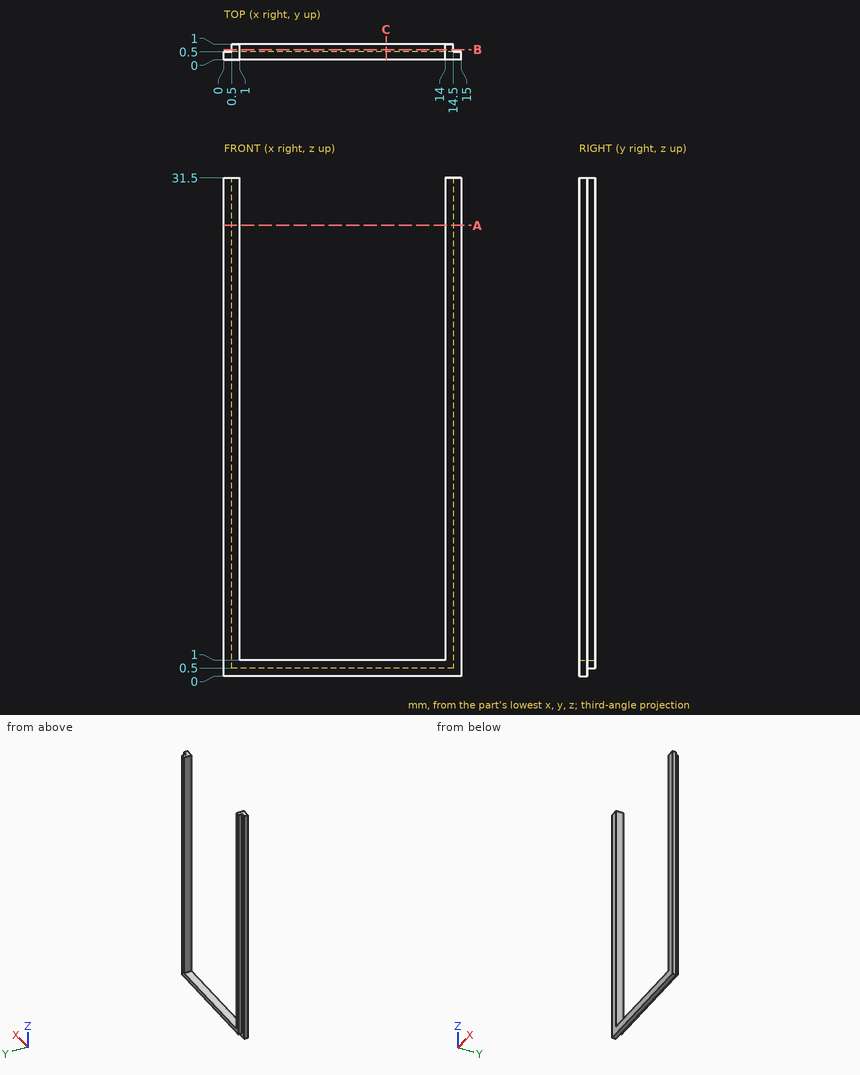
For this review, use the dimensioned drawing (mm, ordinates from the lowest corner) and the shaded views. Give positions to 0.01 mm unless a question says otherwise; leave off trailing zeros. Write each loop counter-clockwise with the first axis right and the second up, starting at its lowest first coordinate (ties: lowest second). Pieces come first, ordered by that corner, then holes.
(1) Consider section C-C, the plane x = 10.25. Give the boundary of the cut face in (y, z).
(2) To check wall thickness, follow L1, parallel to X at y = 0.55, z = 13; L2, parallel to X at y = 0.2, z = 13; L3, parallel to Z at x = 13.25, y = 0.3. State the ranges of each line that lie inside material, in increasing order.
(3) For P1, Ø0.6, axis at y = 0.5, z = 10.5, coming from the -X side; P2, Ø4, axis at x = 10.5, z = 27, coming from the -Y side, all flat-tipped, find the tip position at first contact; note any pin that passes through.
(4) Consider section A-A, the plane z = 28.5. Give the boundary of the cut face in (x, y), and give its area (3 significant figures).
(5) Consider section B-B, the plane y = 0.65. Give the boundary of the cut face in (x, z).
Returned:
1. outline: (0, 0) - (0.5, 0) - (0.5, 0.5) - (1, 0.5) - (1, 1) - (0, 1) - close
2. L1: x = 0.5 to 1, 14 to 14.5
2. L2: x = 0 to 1, 14 to 15
2. L3: z = 0 to 1
3. P1: stops at x = 0
3. P2: passes through
4. outline: (0, 0) - (1, 0) - (1, 1) - (0.5, 1) - (0.5, 0.5) - (0, 0.5) - close; (14, 0) - (15, 0) - (15, 0.5) - (14.5, 0.5) - (14.5, 1) - (14, 1) - close
4. area: 1.50 mm2
5. outline: (0.5, 0.5) - (14.5, 0.5) - (14.5, 31.5) - (14, 31.5) - (14, 1) - (1, 1) - (1, 31.5) - (0.5, 31.5) - close
